CAD build for the part. Positions are in the model's coordinates, mm. Coordinates: 2 decimals unless noted, no trailing zeros. Loops run counter-clockwise (first coordinate to the right, second up) from the corner with the lowest first, then second, coordinate; pieces in that order, holes last. Notation, with made-up numbers: (-38.75, 89) -> (13.25, 89) arc R25 ccw to (13.25, 122) -> close; hole circle Ø9 at (-19, -14.5). An arc over 180 degrees is marked (long way). Answer as a JSON object with one key per item and string values. Group by question number.
from build123d import *

# Parameters (mm, degrees)
SKETCH2_R           = 1.6
BOSS_EXTRUDE3_DEPTH = 1


with BuildPart() as part:
    # Sketch2 → Boss-Extrude3 (new body)
    with BuildSketch(Plane(origin=(0, 0, 0), x_dir=(1, 0, 0), z_dir=(0, 1, 0))):
        with BuildLine():
            Line((-46.858540632, 41.275), (-46.858540632, -41.275))
            ThreePointArc((-46.858540632, -41.275), (-45.557936393, -44.414936393), (-42.418, -45.715540632))
            Line((-42.418, -45.715540632), (42.418, -45.715540632))
            ThreePointArc((42.418, -45.715540632), (45.557936393, -44.414936393), (46.858540632, -41.275))
            Line((46.858540632, -41.275), (46.858540632, 41.275))
            ThreePointArc((46.858540632, 41.275), (45.557936393, 44.414936393), (42.418, 45.715540632))
            Line((42.418, 45.715540632), (22.418, 45.715540632))
            Line((22.418, 45.715540632), (22.418, 41.275))
            Line((22.418, 41.275), (22.418, 39.575))
            Line((22.418, 39.575), (22.418, 37.797317828))
            Line((22.418, 37.797317828), (20.16872062, 37.797317828))
            Line((20.16872062, 37.797317828), (20.16872062, 9.575))
            Line((20.16872062, 9.575), (20.16872062, 7.075))
            Line((20.16872062, 7.075), (21.96872062, 7.075))
            Line((21.96872062, 7.075), (21.96872062, 0.094907102))
            Line((21.96872062, 0.094907102), (-9.912382857, 0.094907102))
            Line((-9.912382857, 0.094907102), (-16.875382857, 0.094907102))
            Line((-16.875382857, 0.094907102), (-16.875382857, 30.218907102))
            Line((-16.875382857, 30.218907102), (-16.875382857, 45.715540632))
            Line((-16.875382857, 45.715540632), (-42.418, 45.715540632))
            ThreePointArc((-42.418, 45.715540632), (-45.557936393, 44.414936393), (-46.858540632, 41.275))
        make_face()
        with Locations(Location((-42.418, -41.275, 0), (0, 0, 270))):
            Circle(SKETCH2_R, mode=Mode.SUBTRACT)
        Polygon((-36.724382857, -36.217092898), (-36.724382857, -29.217092898), (-36.724382857, -22.217092898), (-22.724382857, -22.217092898), (-22.724382857, -36.217092898), align=None, mode=Mode.SUBTRACT)
        Polygon((-16.912382857, -22.217092898), (-9.912382857, -22.217092898), (-2.912382857, -22.217092898), (-2.912382857, -36.217092898), (-16.912382857, -36.217092898), align=None, mode=Mode.SUBTRACT)
        Polygon((-36.724382857, -16.405092898), (-36.724382857, -9.405092898), (-36.724382857, -2.405092898), (-22.724382857, -2.405092898), (-22.724382857, -16.405092898), align=None, mode=Mode.SUBTRACT)
        Polygon((-2.912382857, -16.405092898), (-9.912382857, -16.405092898), (-16.912382857, -16.405092898), (-16.912382857, -2.405092898), (-2.912382857, -2.405092898), align=None, mode=Mode.SUBTRACT)
        Polygon((2.899617143, -22.217092898), (9.899617143, -22.217092898), (16.899617143, -22.217092898), (16.899617143, -36.217092898), (2.899617143, -36.217092898), align=None, mode=Mode.SUBTRACT)
        with Locations(Location((42.418, -41.275, 0), (0, 0, 270))):
            Circle(SKETCH2_R, mode=Mode.SUBTRACT)
        Polygon((36.711617143, -22.217092898), (36.711617143, -29.217092898), (36.711617143, -36.217092898), (22.711617143, -36.217092898), (22.711617143, -22.217092898), align=None, mode=Mode.SUBTRACT)
        Polygon((2.899617143, -2.405092898), (9.899617143, -2.405092898), (16.899617143, -2.405092898), (16.899617143, -16.405092898), (2.899617143, -16.405092898), align=None, mode=Mode.SUBTRACT)
        Polygon((22.711617143, -2.405092898), (29.711617143, -2.405092898), (36.711617143, -2.405092898), (36.711617143, -16.405092898), (22.711617143, -16.405092898), align=None, mode=Mode.SUBTRACT)
        Polygon((-38.375382857, 3.406907102), (-38.375382857, 10.406907102), (-38.375382857, 17.406907102), (-24.375382857, 17.406907102), (-24.375382857, 3.406907102), align=None, mode=Mode.SUBTRACT)
        Polygon((-46.218, 27.292), (-46.218, 28.892), (-46.218, 30.492), (-38.375382857, 30.492), (-38.375382857, 37.218907102), (-31.375382857, 37.218907102), (-24.375382857, 37.218907102), (-24.375382857, 23.218907102), (-38.375382857, 23.218907102), (-38.375382857, 27.292), align=None, mode=Mode.SUBTRACT)
        with Locations(Location((-42.418, 41.275, 0), (0, 0, 270))):
            Circle(SKETCH2_R, mode=Mode.SUBTRACT)
        Polygon((38.362617143, 17.406907102), (38.362617143, 10.406907102), (38.362617143, 3.406907102), (24.362617143, 3.406907102), (24.362617143, 17.406907102), align=None, mode=Mode.SUBTRACT)
        Polygon((46.218, 27.292), (42.418, 27.292), (38.362617143, 27.292), (38.362617143, 23.218907102), (24.362617143, 23.218907102), (24.362617143, 37.218907102), (38.362617143, 37.218907102), (38.362617143, 30.492), (42.418, 30.492), (46.218, 30.492), align=None, mode=Mode.SUBTRACT)
        with Locations(Location((42.418, 41.275, 0), (0, 0, 270))):
            Circle(SKETCH2_R, mode=Mode.SUBTRACT)
    extrude(amount=BOSS_EXTRUDE3_DEPTH)


solid = part.part
Item 1: Band-saw the part on A-A, the plane z = -25. List the corners of the cut face in (x, y), and give its area (3 significant figures).
Item 2: Band-saw the part on C-C, the plane z = 31.5. List the corners of the cut face in (x, y), and give its area (3 significant figures).
Item 3: Pull direction Z, two halves, no side cores. Call faces 1 (the cylindrical face through (-40.83, 0.49, -41.48)), 2 (the cylindrical face through (-45.59, 0.49, 44.38)), 3 (the cylindrical face through (45.59, 0.49, -44.38)): +Z half, -Z half, draft (parallel to the pull), parting line (faces both ways), or undercut.
Item 4: Band-saw the part on B-B, the plane x = -11. List the corners of the cut face in (y, z), and give its area (3 significant figures).
Item 5: Drill centre lines: L1, parallel to X at y = 0.8, z = 16; L2, parallel to X at y = 0.3, z = -3.5; L3, parallel to Z at x = -5.5, y = 0.9. Where is each one in solid material? Low to high.
Item 6: Band-saw the part on D-D, the plane x = 26.5. List the corners of the cut face in (y, z).
Reply:
{
 "1": {"outline": "(-46.86, 0) -> (-38.38, 0) -> (-38.38, 1) -> (-46.86, 1) -> close; (-24.38, 0) -> (-16.88, 0) -> (-16.88, 1) -> (-24.38, 1) -> close; (20.17, 0) -> (24.36, 0) -> (24.36, 1) -> (20.17, 1) -> close; (38.36, 0) -> (46.86, 0) -> (46.86, 1) -> (38.36, 1) -> close", "area": "28.7 mm²"},
 "2": {"outline": "(-46.86, 0) -> (-36.72, 0) -> (-36.72, 1) -> (-46.86, 1) -> close; (-22.72, 0) -> (-16.91, 0) -> (-16.91, 1) -> (-22.72, 1) -> close; (-2.91, 0) -> (2.9, 0) -> (2.9, 1) -> (-2.91, 1) -> close; (16.9, 0) -> (22.71, 0) -> (22.71, 1) -> (16.9, 1) -> close; (36.71, 0) -> (46.86, 0) -> (46.86, 1) -> (36.71, 1) -> close", "area": "37.7 mm²"},
 "3": {"face 1": "undercut", "face 2": "+Z half", "face 3": "-Z half"},
 "4": {"outline": "(0, -0.09) -> (1, -0.09) -> (1, 2.41) -> (0, 2.41) -> close; (0, 16.41) -> (1, 16.41) -> (1, 22.22) -> (0, 22.22) -> close; (0, 36.22) -> (1, 36.22) -> (1, 45.72) -> (0, 45.72) -> close", "area": "17.8 mm²"},
 "5": {"L1": "-46.86 to -36.72, -22.72 to -16.91, -2.91 to 2.9, 16.9 to 22.71, 36.71 to 46.86", "L2": "-46.86 to -38.38, -24.38 to -16.88, 21.97 to 24.36, 38.36 to 46.86", "L3": "-0.09 to 2.41, 16.41 to 22.22, 36.22 to 45.72"},
 "6": {"outline": "(0, -45.72) -> (1, -45.72) -> (1, -37.22) -> (0, -37.22) -> close; (0, -23.22) -> (1, -23.22) -> (1, -17.41) -> (0, -17.41) -> close; (0, -3.41) -> (1, -3.41) -> (1, 2.41) -> (0, 2.41) -> close; (0, 16.41) -> (1, 16.41) -> (1, 22.22) -> (0, 22.22) -> close; (0, 36.22) -> (1, 36.22) -> (1, 45.72) -> (0, 45.72) -> close"}
}
